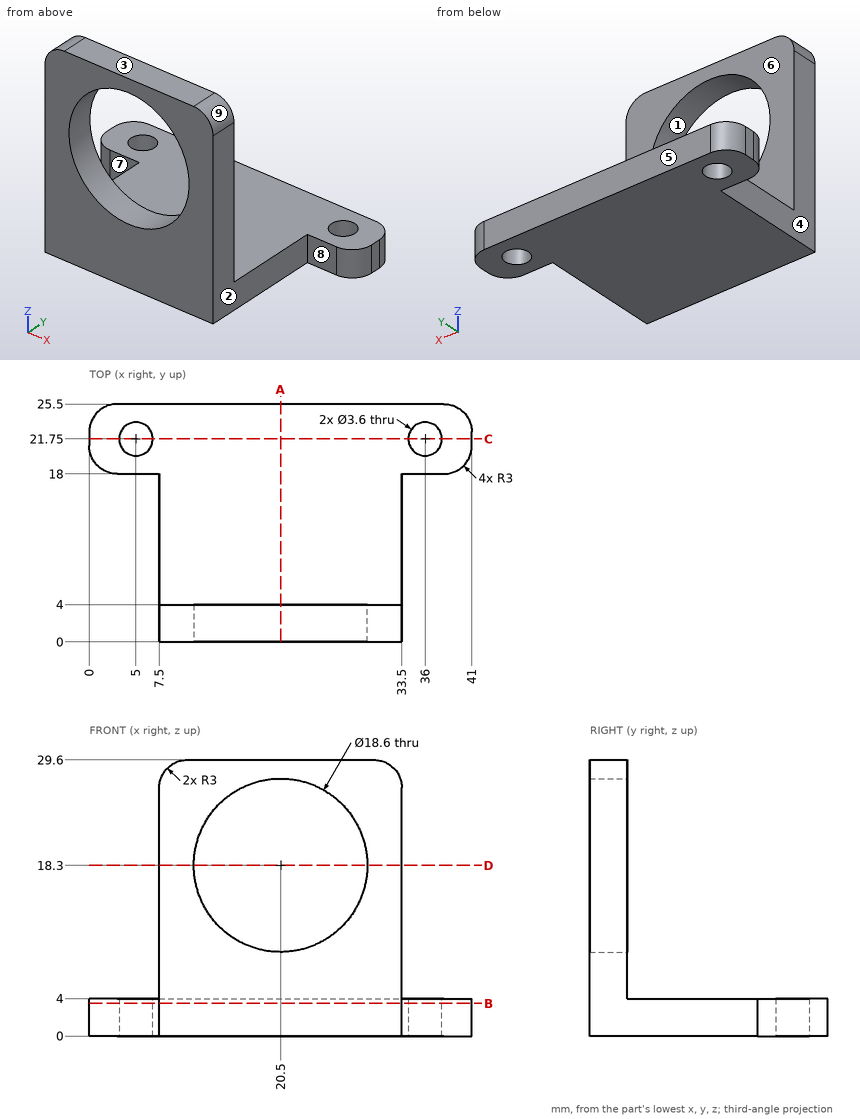
The figure shows three views and two pictorial views of one solid part (mm, origin at its lowest corner). Answer the questions. A direction names the side the tool comes from. Coordinates: 2 decimals unless noted, no trailing zeros. Loops run counter-clockwise (first coordinate to the right, second up) from the corner with the lowest first, then second, coordinate; pieces in that order, holes last. Notation, with made-up numbers: (59.5, -13) - (63.5, -13) arc R19 ccw to (63.5, 19) - close; hole circle Ø9 at (25, 34.5). An arc over 180 degrees is marked (long way). Answer in a Markdown table with one row per item.
Q1. For the marked faces 5, 6, 7, 8 and 9, determine the directions among +Z, -Z, +X, -X, +Y, -Y from which every point of the face is accessible in a straight line to the end or side of a thin tool.
Here are the results:
| item | result |
|---|---|
| face 5 | +Z, -Z, +X, -X, +Y |
| face 6 | +Z, +X, -X, +Y |
| face 7 | +Z, -Z, -X, -Y |
| face 8 | +Z, -Z, +X, -Y |
| face 9 | +Z, +X, +Y, -Y |
Q2. Find section B-B on z = 3.5. Write down the section's boundary in (x, y).
Here are the results:
| item | result |
|---|---|
| outline | (0, 21) arc R3 ccw to (3, 18) - (7.5, 18) - (7.5, 0) - (33.5, 0) - (33.5, 18) - (38, 18) arc R3 ccw to (41, 21) - (41, 22.5) arc R3 ccw to (38, 25.5) - (3, 25.5) arc R3 ccw to (0, 22.5) - close; hole circle Ø3.6 at (5, 21.75); hole circle Ø3.6 at (36, 21.75) |
Q3. Given P1, Ø5.5, axis at y = 6, z = 12, coming from the -X side; P2, Ø2, axis at x = 4.5, z = 2, coming from the -Y side; P3, Ø14.5, axis at y = 7, z = 16.5, coming from the +X side, each flat-ended and moving along its own axis, determine where each tip first touches the part or whether it passes through.
Here are the results:
| item | result |
|---|---|
| P1 | stops at x = 7.5 |
| P2 | stops at y = 18 |
| P3 | stops at x = 33.5 |
Q4. Find section D-D on z = 18.3. Write down the section's boundary in (x, y), plus the area to 3 significant figures.
Here are the results:
| item | result |
|---|---|
| outline | (7.5, 0) - (11.2, 0) - (11.2, 4) - (7.5, 4) - close; (29.8, 0) - (33.5, 0) - (33.5, 4) - (29.8, 4) - close |
| area | 29.6 mm^2 |
Q5. Straight lines are drawn through the part: line 1 along Y through (x, z) = (36, 1.85); line 2 along Z through (x, y) = (20.5, 2); line 3 along Y through (x, z) = (32, 13.75). For each, find the intervals that lie inside material, in ascending order. Write a range as [from, to].
Here are the results:
| item | result |
|---|---|
| line 1 | y = [18, 19.95], [23.55, 25.5] |
| line 2 | z = [0, 9], [27.6, 29.6] |
| line 3 | y = [0, 4] |
Q6. Find section C-C on y = 21.75. Write down the section's boundary in (x, z), plus the area to 3 significant figures.
Here are the results:
| item | result |
|---|---|
| outline | (0, 0) - (3.2, 0) - (3.2, 4) - (0, 4) - close; (6.8, 0) - (34.2, 0) - (34.2, 4) - (6.8, 4) - close; (37.8, 0) - (41, 0) - (41, 4) - (37.8, 4) - close |
| area | 135 mm^2 |
Q7. The mould has two halves that part along X. Classify the marked faces 1, 2, 3 and 4: pulls with the +X half, pulls with the -X half, needs draft (parallel to the pull), parting line crosses it, or undercut.
Here are the results:
| item | result |
|---|---|
| face 1 | undercut |
| face 2 | pulls with the +X half |
| face 3 | needs draft |
| face 4 | pulls with the -X half |
Q8. Find section A-A on x = 20.5. Write down the section's boundary in (y, z).
Here are the results:
| item | result |
|---|---|
| outline | (0, 0) - (25.5, 0) - (25.5, 4) - (4, 4) - (4, 9) - (0, 9) - close; (0, 27.6) - (4, 27.6) - (4, 29.6) - (0, 29.6) - close |
